Here's how the part is built. I have some questions about the finished solid (model axes, mm). Face numbers are marked on the shaded views. A direction names the side the tool comes from. Give positions to 0.01 mm unless a question says otherwise; leave off trailing zeros. Loops run counter-clockwise (first coordinate to the right, second up) from the corner with the lowest first, then second, coordinate; pieces in that order, holes last.
Q1. Suppose I cut it at D-D (y = -1.5). List the corners of the cut face in (x, z) for me.
Q2. I need wall thicknesses on probe 1 along Z at (x, y) = (-57, 1.1); probe 2 along Y at (x, z) = (-55.75, -7); probe 3 along X at (y, z) = (-1.4, -7). Which ranges of each line are inside material? Lowest first, please.
Q3. Suppose I cut it at C-C (x = -52.75). List the corners of the cut face in (y, z) for me (3 decimals), and give its area (3 significant figures).
Q4. I'm going to push flat-ended pins straight in: P1, Ø0.5, axis at x = -56, z = -2, coming from the -Y side; P2, Ø1.3, axis at x = -54.5, z = -4.5, coming from the +Y side; P3, Ø0.7, axis at x = -55, z = -1.5, coming from the -Y side. Where does each tip first touch, or does it pass through?
Q5. Thinking about a two-plate mould opening in X: for the marked faces 4, 5 and 6, which applies, pulls with the +X half, pulls with the -X half, needs draft (parallel to the pull), parting line crosses it, or undercut?
Q6. Suppose I cut it at A-A (y = 0). List the corners of the cut face in (x, z) for me.
Q7. For the marked faces 1, 2 and 3, which set-ups out of +Z, -Z, +X, -X, +Y, -Y let a thin tool reach every point of the face, with its end or its side?
Q8. Suppose I cut it at B-B (z = 2). List the corners of the cut face in (x, y) for me, and give its area (3 significant figures).
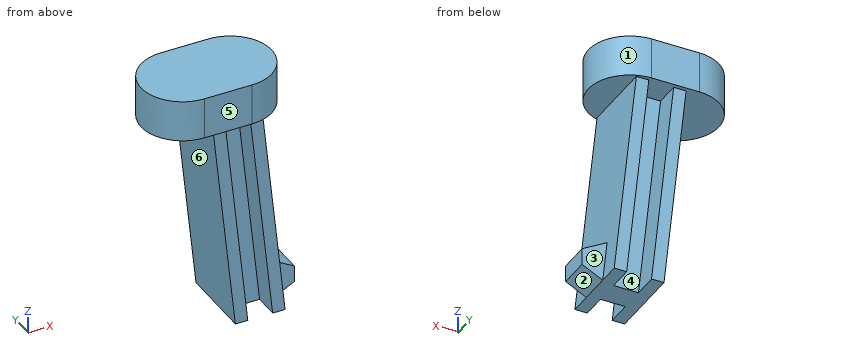
```python
from build123d import *

# Parameters (mm, degrees)
PAD005_DEPTH    = 1.8
POCKET004_DEPTH = 1.2
PAD007_DEPTH    = 2
PAD011_DEPTH    = 0.75


with BuildPart() as part:
    # Sketch008 → Pad005 (new body, symmetric)
    with BuildSketch(Plane.XZ):
        Polygon((-53.3, -8.3), (-54.367859, 1.86), (-56.767859, 1.86), (-55.7, -8.3), align=None)
    extrude(amount=PAD005_DEPTH, both=True)

    # Sketch010 (on DatumPlane) → Pocket004 (cut)
    with BuildSketch(Plane.XZ.offset(1.8)):
        Polygon((-53.9, -8.3), (-54.967859, 1.86), (-56.167859, 1.86), (-55.1, -8.3), align=None)
    pocket004 = extrude(amount=-POCKET004_DEPTH, mode=Mode.SUBTRACT)

    # Mirrored002: Pocket004 across XZ
    add(pocket004.mirror(Plane.XZ), mode=Mode.SUBTRACT)

    # Sketch014 (on DatumPlane) → Pad007 (join)
    with BuildSketch(Plane.XY.offset(1.86)):
        with BuildLine():
            ThreePointArc((-57.3, 2), (-59.3, 0), (-57.3, -2))
            Line((-57.3, -2), (-55, -2))
            ThreePointArc((-55, -2), (-53, 0), (-55, 2))
            Line((-57.3, 2), (-55, 2))
        make_face()
    extrude(amount=PAD007_DEPTH)

    # Sketch023 → Pad011 (join, symmetric)
    with BuildSketch(Plane.XZ):
        Polygon((-53.509057, -6.310956), (-53.3, -8.3), (-52.3, -7.8), (-52.3, -7), align=None)
    extrude(amount=PAD011_DEPTH, both=True)


solid = part.part
```
Solutions:
1. outline: (-58.62, 1.86) - (-56.77, 1.86) - (-55.7, -8.3) - (-55.1, -8.3) - (-56.17, 1.86) - (-54.97, 1.86) - (-53.9, -8.3) - (-53.3, -8.3) - (-54.37, 1.86) - (-53.68, 1.86) - (-53.68, 3.86) - (-58.62, 3.86) - close
2. probe 1: z = 1.86 to 3.86
2. probe 2: y = -1.8 to 1.8
2. probe 3: x = -55.84 to -55.24, -54.04 to -53.44
3. outline: (-0.75, -8.025) - (0.75, -8.025) - (0.75, -6.744) - (-0.75, -6.744) - close
3. area: 1.92 mm2
4. P1: stops at y = -1.8
4. P2: stops at y = 1.8
4. P3: stops at y = -0.6
5. face 4: undercut
5. face 5: needs draft
5. face 6: pulls with the -X half
6. outline: (-59.3, 1.86) - (-56.77, 1.86) - (-55.7, -8.3) - (-53.3, -8.3) - (-52.3, -7.8) - (-52.3, -7) - (-53.51, -6.31) - (-54.37, 1.86) - (-53, 1.86) - (-53, 3.86) - (-59.3, 3.86) - close
7. face 1: +Z, +X
7. face 2: -Z, +X, +Y, -Y
7. face 3: +X, +Y
8. outline: (-57.3, -2) - (-55, -2) arc R2 ccw to (-55, 2) - (-57.3, 2) arc R2 ccw to start
8. area: 21.8 mm2
